Check sheet for the modelled part. Datum: model origin and axes. Units: mm. Face numbers are marked on the shaded views. A direction names the side the tool comes from. Round coordinates to 2 decimals unless told otherwise and drop trailing zeros. Order: outer loops, then holes, each group sorted by start corner. A loop starts at its lowest first (then second) coordinate and runs counter-clockwise, first axis right, second up. Notation, with made-up numbers: M -14,28 L 16,28 A21 ccw 16,45 Z; hole C 76.5,3.25 d5. An arc over 180 degrees is marked long. One line per item, written item: value. Start each with the question number.
(1) Cross-section at D-D, the plane y = 2.5. Enter the section's corners in (x, z).
(2) Access from +Z, -Z, +X, -X, +Y, -Y to the whole of each face (thin tool, end or side, straight path). Record for the marked faces 5 and 6.
(3) Cross-section at C-C, the plane x = 17.5. Enter the section's corners in (y, z), and give its area (3 significant figures).
(4) Cross-section at B-B, the plane z = 0.7. Enter the section's corners in (x, y), and give its area (3 significant figures).
(5) Release check for a two-part mould opening along Y. For the marked faces 1, 2, 3 and 4 record: released by +Y, released by -Y, zero draft, split by the parting line, or undercut.
(6) Thickness scan on L1, parallel to Y at x = 17, z = 1.05; L2, parallel to X at y = 0.25, z = 1.5; L3, parallel to X at y = 0.75, z = 1.05. Record the ranges inside material, lowest first.
(7) Depth check by flat-ended pin: pin 1 Ø3 at (x, y) = (10.5, -2) entering from -Z. Enter the tip coordinate at first touch or a pass-through.
(8) Cross-section at A-A, the plane y = 0. Enter the section's corners in (x, z).
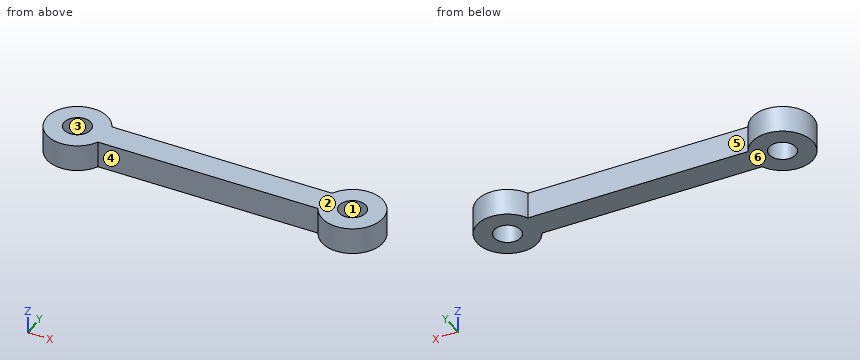
from build123d import *

# Parameters (mm, degrees)
SKETCH2_R           = 3.436597574
SKETCH2_R_2         = 1.5
BOSS_EXTRUDE1_DEPTH = 3


with BuildPart() as part:
    # Sketch2 → Boss-Extrude1 (new body)
    # profile 1 of 3: a face of its own
    with BuildSketch(Plane.XY):
        with Locations((-14.105820106, 0)):
            Circle(SKETCH2_R)
        with Locations((-14.105820106, 0)):
            Circle(SKETCH2_R_2, mode=Mode.SUBTRACT)
    # profile 2 of 3: a face of its own
    with BuildSketch(Plane.XY):
        with BuildLine():
            Line((13.802222119, 1.5), (-11.01386233, 1.5))
            ThreePointArc((-11.01386233, 1.5), (-10.756490511, 0.769541518), (-10.669222532, 0))
            ThreePointArc((-10.669222532, 0), (-10.756490511, -0.769541518), (-11.01386233, -1.5))
            Line((-11.01386233, -1.5), (13.802222119, -1.5))
            ThreePointArc((13.802222119, -1.5), (13.45758232, 0), (13.802222119, 1.5))
        make_face()
    # profile 3 of 3: a face of its own
    with BuildSketch(Plane.XY):
        with Locations((16.894179894, 0)):
            Circle(SKETCH2_R)
        with Locations((16.894179894, 0)):
            Circle(SKETCH2_R_2, mode=Mode.SUBTRACT)
    extrude(amount=BOSS_EXTRUDE1_DEPTH)


solid = part.part
Values found:
1. outline: M -16.46,0 L -11.75,0 L -11.75,3 L -16.46,3 Z; M 14.54,0 L 19.25,0 L 19.25,3 L 14.54,3 Z
2. face 5: +Z, -Z, +Y
2. face 6: -Z, +X, -X, +Y, -Y
3. outline: M -3.38,0 L -1.37,0 L -1.37,3 L -3.38,3 Z; M 1.37,0 L 3.38,0 L 3.38,3 L 1.37,3 Z
3. area: 12.1 mm^2
4. outline: M -11.01,-1.5 L 13.8,-1.5 A3.44 ccw long 13.8,1.5 L -11.01,1.5 A3.44 ccw long Z; hole C -14.11,0 d3; hole C 16.89,0 d3
4. area: 133 mm^2
5. face 1: undercut
5. face 2: zero draft
5. face 3: undercut
5. face 4: released by -Y
6. L1: -3.43 to -1.5, 1.5 to 3.43
6. L2: -17.53 to -15.58, -12.63 to 15.42, 18.37 to 20.32
6. L3: -17.46 to -15.4, -12.81 to 15.6, 18.19 to 20.25
7. pin 1: z = 0
8. outline: M -17.54,0 L -15.61,0 L -15.61,3 L -17.54,3 Z; M -12.61,0 L 15.39,0 L 15.39,3 L -12.61,3 Z; M 18.39,0 L 20.33,0 L 20.33,3 L 18.39,3 Z
